Geometry: final body of the model. Coordinates: model frame, mm. Face numbers are marked on the shaded views. A direction names the side the tool comes from. Give positions to 0.01 mm unless a question says otherwise; leave off trailing zeros. Loops run counter-clockwise (first coordinate to the right, second up) from the corner with the lowest first, then second, coordinate; pieces in that order, holes last. Notation, with made-up numbers: (27, 82.25) -> (39, 82.25) arc R25 ccw to (39, 100.25) -> close; hole circle Ø4 at (-17.75, 64). An arc over 180 degrees is marked (long way). Answer in a Markdown table with one row per item. Add a question column.
1) Section query A-A (x = 15.5). Return the cut outline in (y, z).
2) First-contact query: P1, Ø3.5, axis at y = 22, z = -11, coming from the -X side; P2, Ø3, axis at x = -29, y = 28.5, coming from the -Z side; P3, Ø10, axis at y = 8.5, z = 0.5, coming from the -X side. Flat tips, straight axial feed; report the tip coordinate or a pass-through.
3) Access query for the marked faces 1 and 2. Directions: +Z, -Z, +X, -X, +Y, -Y. A direction counts if a zero-diameter tool reaches every point of the face in a straight line with its end or side. Return the directions, or none.
4) Section query C-C (y = -26). Return the cut outline in (x, z), plus the area to 3 significant figures.
5) Line query: line 1 (Y direction, x = 7.5, z = -9); line 2 (Y direction, x = 28, z = -10.75); line 3 (Y direction, x = -11, z = -1.5). Output: solid intervals per line, ascending. Write a range as from..to.
6) Section query D-D (x = -4). Return the cut outline in (y, z), plus the area to 3 significant figures.
7) Section query B-B (z = 7.5). Return the cut outline in (x, y).
Autodesk Inventor part; units mm, degrees
ref_plane "Work Plane1" through (-95.3031, 23.4838, 9.5) normal (0, 0, -1) x (-0.001, 1, 0)
ref_plane "YZ Plane" through (0, 0, 0) normal (1, 0, 0) x (0, 1, 0)
ref_plane "XZ Plane" through (0, 0, 0) normal (0, 1, 0) x (-1, 0, 0)
sketch "Sketch1" plane through (0, 0, 0) normal (0, 0, 1) x (1, 0, 0)
  circle A0 centre (-31.2153, 30.6223) radius 1.5
  line L0 (22.8696, 23.547) -> (22.8696, 28.547)
  line L1 (-24.2436, 23.547) -> (22.8696, 23.547)
  line L2 (-24.2436, 23.547) -> (-29.0502, 31.8723)
  arc A1 (-29.0502, 31.8723) -> (-33.3804, 29.3723) centre (-31.2153, 30.6223) ccw
  line L3 (-33.3804, 29.3723) -> (-27.1304, 18.547)
  line L4 (27.8696, 18.547) -> (-27.1304, 18.547)
  line L5 (27.8696, -36.453) -> (27.8696, 18.547)
  line L6 (-2.1304, -36.453) -> (27.8696, -36.453)
  line L7 (2.8696, -41.453) -> (-2.1304, -36.453)
  line L8 (32.8696, -41.453) -> (2.8696, -41.453)
  line L9 (32.8696, 28.547) -> (32.8696, -41.453)
  arc A2 (32.8696, 28.547) -> (22.8696, 28.547) centre (27.8696, 28.547) ccw
  line L10 (27.8696, 18.547) -> (-27.1304, 18.547)
  line L11 (-24.2436, 23.547) -> (-27.1304, 23.547)
  line L12 (-27.1304, 18.547) -> (-27.1304, 23.547)
  line L13 (-27.1304, 23.547) -> (-24.2436, 23.547)
  line L14 (-24.2436, 23.547) -> (32.8696, 23.547)
  line L15 (32.8696, 28.547) -> (32.8696, -41.453)
  point P0 (0, 0)
  point P1 (-2.3882, 28.0958)
  point P2 (32.8696, 23.547)
  point P3 (22.8696, 23.547)
  dimension "d6" = 10
  dimension "d7" = 60
  dimension "d9" = 30
  dimension "d10" = 55
  dimension "d11" = 5
  dimension "d14" = 65
  dimension "d15" = 5
  dimension "d19" = 5
  dimension "d20" = 5
  dimension "d28" = 30
extrude "Extrusion1" add sketch "Sketch1" along normal mid plane 25 contours L14 L9 L8 L7 L6 L5 L4 L12 L11 L1
extrude "Extrusion2" add sketch "Sketch1" along normal mid plane 19 contours L11 L12 L3 A1 L2
extrude "Extrusion3" cut sketch "Sketch1" along normal mid plane 13 contours L0 A2 L9 L14 | L11 L12 L3 A1 L2
ref_plane "Work Plane1" through (-95.3031, 23.4838, 9.5) normal (0, 0, -1) x (-0.001, 1, 0)
extrude "Extrusion5" add sketch "Sketch1" along normal mid plane 19 contours L0 A2 L9 L14
extrude "Extrusion6" cut sketch "Sketch1" along normal mid plane 13 contours L0 A2 L9 L14
sketch "Sketch3" plane through (0, 0, 9.5) normal (0, 0, 1) x (1, 0, 0)
  arc A0 (32.8696, 28.547) -> (22.8696, 28.547) centre (27.8696, 28.547) ccw
  circle A1 centre (27.8696, 28.547) radius 2.5
  point P0 (0, 0)
  dimension "d25" = 5
extrude "Extrusion7" cut sketch "Sketch3" against normal through all
properties part number "Claw New side"
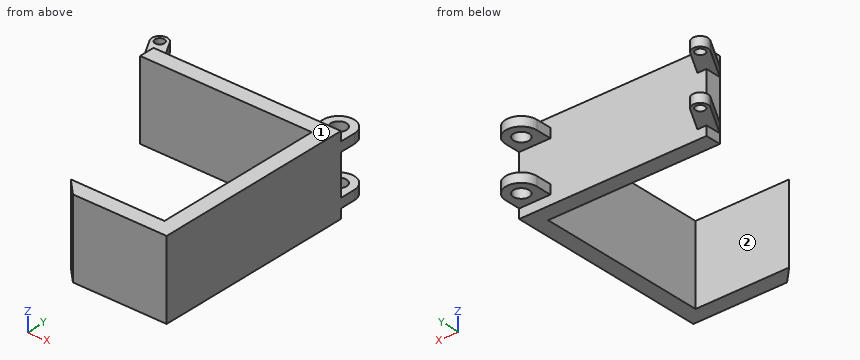
Evaluation:
| question | item | result |
|---|---|---|
| 1 | outline | (-41.45, -12.5) -> (-36.45, -12.5) -> (-36.45, 12.5) -> (-41.45, 12.5) -> close; (18.55, -12.5) -> (23.55, -12.5) -> (23.55, 12.5) -> (18.55, 12.5) -> close |
| 2 | P1 | x = -29.64 |
| 2 | P2 | z = -9.5 |
| 2 | P3 | x = 27.87 |
| 3 | face 1 | +Z, +X, -X, +Y, -Y |
| 3 | face 2 | +Z, -Z, -X |
| 4 | outline | (27.87, -12.5) -> (32.87, -12.5) -> (32.87, 12.5) -> (27.87, 12.5) -> close |
| 4 | area | 125 mm² |
| 5 | line 1 | -41.45..-36.45, 18.55..23.55 |
| 5 | line 2 | -41.45..23.55 |
| 5 | line 3 | 18.55..23.55 |
| 6 | outline | (18.55, -12.5) -> (23.55, -12.5) -> (23.55, 12.5) -> (18.55, 12.5) -> close |
| 6 | area | 125 mm² |
| 7 | outline | (-33.38, 29.37) -> (-27.13, 18.55) -> (27.87, 18.55) -> (27.87, -36.45) -> (-2.13, -36.45) -> (2.87, -41.45) -> (32.87, -41.45) -> (32.87, 28.55) arc R5 ccw to (22.87, 28.55) -> (22.87, 23.55) -> (-24.24, 23.55) -> (-29.05, 31.87) arc R2.5 ccw to start; hole circle Ø3 at (-31.22, 30.62); hole circle Ø5 at (27.87, 28.55) |
